from build123d import *

# Parameters (mm, degrees)
SKETCH1_W                    = 25
SKETCH1_H                    = 50
BASE_FLANGE1_DEPTH           = 3.175
EDGE_FLANGE1_STRIP_W         = 19.05
EDGE_FLANGE1_STRIP_H         = 3.175
EDGE_FLANGE1_STRIP_CUT_DEPTH = 25
EDGE_FLANGE1_DEPTH           = 25
M12_CLEARANCE_HOLE1_D        = 13.5
M4_CLEARANCE_HOLE1_D         = 4.5
FILLET1_R                    = 10
FILLET2_R                    = 2


# Sheet-metal steps are written as plain solids
with BuildPart() as part:
    # Sketch1 → Base-Flange1 (new body)
    with BuildSketch(Plane(origin=(0, 0, 0), x_dir=(1, 0, 0), z_dir=(0, 1, 0))):
        with Locations((0, 25)):
            Rectangle(SKETCH1_W, SKETCH1_H)
    extrude(amount=-BASE_FLANGE1_DEPTH)

    # Edge-Flange1 strip (across the edge) → Edge-Flange1 strip cut (cut)
    with BuildSketch(Plane(origin=(12.5, 0, -50), x_dir=(0, 0, 1), z_dir=(-1, 0, 0))):
        with Locations((-3.175, -1.5875)):
            Rectangle(EDGE_FLANGE1_STRIP_W, EDGE_FLANGE1_STRIP_H)
    extrude(amount=EDGE_FLANGE1_STRIP_CUT_DEPTH, mode=Mode.SUBTRACT)

    # Edge-Flange1 section (across the edge) → Edge-Flange1 (add)
    with BuildSketch(Plane(origin=(12.5, 0, -50), x_dir=(0, 0, 1), z_dir=(-1, 0, 0))):
        with BuildLine():
            Line((0, 3.175), (0, 23.825))
            Line((0, 23.825), (3.175, 23.825))
            Line((3.175, 23.825), (3.175, 3.175))
            ThreePointArc((3.175, 3.175), (4.10493597, 0.92993597), (6.35, 0))
            Line((6.35, 0), (6.35, -3.175))
            ThreePointArc((6.35, -3.175), (1.859871939, -1.315128061), (0, 3.175))
        make_face()
    extrude(amount=EDGE_FLANGE1_DEPTH)

    # M12 Clearance Hole1 (through all)
    with Locations(Plane(origin=(0, 0, -50), x_dir=(-1, 0, 0), z_dir=(0, 0, -1))):
        with Locations((0, 13.5)):
            Hole(M12_CLEARANCE_HOLE1_D / 2)

    # M4 Clearance Hole1 (through all)
    with Locations(Plane(origin=(0, 0, 0), x_dir=(1, 0, 0), z_dir=(0, 1, 0))):
        with Locations((-7.5, 5), (7.5, 38.65)):
            Hole(M4_CLEARANCE_HOLE1_D / 2)

    # Fillet1
    fillet1_edges = [part.edges().sort_by_distance(p)[0] for p in [
        (12.5, 23.825, -48.4125),
        (-12.5, 23.825, -48.4125),
    ]]
    fillet(fillet1_edges, radius=FILLET1_R)

    # Fillet2
    fillet2_edges = [part.edges().sort_by_distance(p)[0] for p in [
        (12.5, -1.5875, 0),
        (-12.5, -1.5875, 0),
    ]]
    fillet(fillet2_edges, radius=FILLET2_R)


solid = part.part
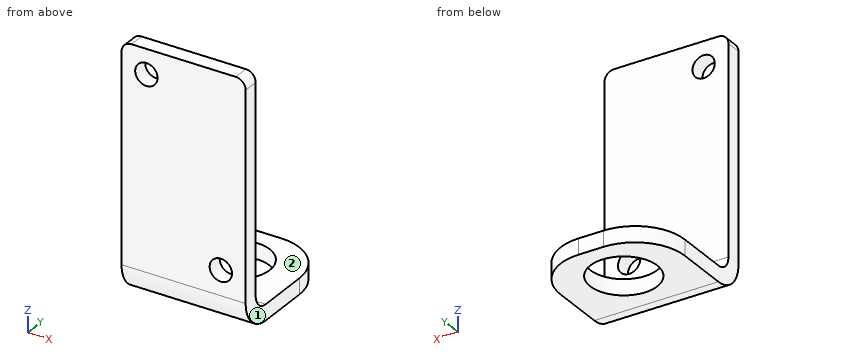
Verification items for the finished model (mm, model axes). Face numbers are marked on the shaded views. A direction names the side the tool comes from. Coordinates: 2 decimals unless noted, no trailing zeros. Loops run counter-clockwise (first coordinate to the right, second up) from the corner with the lowest first, then second, coordinate; pieces in that order, holes last. Notation, with made-up numbers: (11.25, 68.25) -> (24.25, 68.25) arc R18 cw to (24.25, 88.25) -> close; hole circle Ø11 at (86, 86.25). An arc over 180 degrees is marked (long way). Answer as CSV lines item,"result".
1) Thickness scan on L1, parallel to X at y = -1.2, z = -38.65; L2, parallel to Y at x = 10.75, z = -36 (3 decimals); L3, parallel to X at y = -0.5, z = -5.5. Record the ranges inside material, lowest first. Write a range as from..to.
Found:
L1,"x = -12.5..5.25, 9.75..12.5"
L2,"y = -3.175..0"
L3,"x = -12.5..-9.69, -5.31..12.5"
2) Cross-section at A-A, the plane x = 0. Record the cut outline in (y, z) (3 decimals).
Found:
outline,"(-3.175, -43.65) arc R6.35 ccw to (3.175, -50) -> (6.75, -50) -> (6.75, -46.825) -> (3.175, -46.825) arc R3.175 cw to (0, -43.65) -> (0, 0) -> (-3.175, 0) -> close; (20.25, -50) -> (23.825, -50) -> (23.825, -46.825) -> (20.25, -46.825) -> close"
3) Tool access check on the marked faces 1 and 2. Record the directions out of +Z, -Z, +X, -X, +Y, -Y that give a thin tool (end or side, any length) a straight path to the whole face; none if there is none.
Found:
face 1,"+Z, -Z, +X, +Y, -Y"
face 2,"+Z, +X, -X, +Y"
4) Depth check by flat-ended pin: pin 1 (2 mm diameter, centred on x = 8, z = -15, fed in from +Y); pin 2 (10 mm diameter, centred on y = 7.5, z = -32, fed in from +X); pin 3 (10.5 mm diameter, centred on x = -0.5, y = 16.5, fed in from +Z) (3 decimals). Enter the tip coordinate at first touch or a pass-through.
Found:
pin 1,"stops at y = 0"
pin 2,"passes through"
pin 3,"stops at z = -46.825"
5) Cross-section at C-C, the plane y = 12.5. Record the cut outline in (x, z) (3 decimals).
Found:
outline,"(-12.5, -50) -> (-6.676, -50) -> (-6.676, -46.825) -> (-12.5, -46.825) -> close; (6.676, -50) -> (12.5, -50) -> (12.5, -46.825) -> (6.676, -46.825) -> close"
6) Cross-section at B-B, the plane z = -38.65. Record the cut outline in (x, y) (3 decimals), then the cut area to 3 significant figures.
Found:
outline,"(-12.5, -3.175) -> (5.25, -3.175) -> (5.25, 0) -> (-12.5, 0) -> close; (9.75, -3.175) -> (12.5, -3.175) -> (12.5, 0) -> (9.75, 0) -> close"
area,"65.1 mm2"
7) Cross-section at D-D, the plane x = 11.25. Record the cut outline in (y, z) (3 decimals).
Found:
outline,"(-3.175, -43.65) arc R6.35 ccw to (3.175, -50) -> (18.666, -50) -> (18.666, -46.825) -> (3.175, -46.825) arc R3.175 cw to (0, -43.65) -> (0, -0.146) -> (-3.175, -0.146) -> close"
